from build123d import *

# Parameters (mm, degrees)
SKETCH1_W           = 8
SKETCH1_H           = 8
BOSS_EXTRUDE1_DEPTH = 8
BOSS_EXTRUDE2_DEPTH = 6
SKETCH3_OUTSIDE_W   = 19.406
SKETCH3_OUTSIDE_H   = 19.406
SKETCH3_OUTSIDE_W_2 = 10.7
SKETCH3_OUTSIDE_H_2 = 10.7
CUT_EXTRUDE2_DEPTH  = 13.354246922
CHAMFER1_SIZE       = 0.5
CHAMFER1_SIZE2      = 1.37373871
FILLET2_R           = 5
SKETCH6_W           = 8
SKETCH6_H           = 4
CUT_EXTRUDE4_DEPTH  = 12.011130732
MIRROR1_DEPTH       = 6
CUT_EXTRUDE5_DEPTH  = 10.656345064


# Read off the part's stored shape, not the designer's step: Mirror1
with BuildPart() as part:
    # Sketch1 → Boss-Extrude1 (new body)
    with BuildSketch(Plane(origin=(0, 0, 0), x_dir=(1, 0, 0), z_dir=(0, 1, 0))):
        Polygon((6.656854249, -2.757359313), (6.656854249, 2.757359313), (2.757359313, 6.656854249), (-2.757359313, 6.656854249), (-6.656854249, 2.757359313), (-6.656854249, -2.757359313), (-2.757359313, -6.656854249), (2.757359313, -6.656854249), align=None)
        Rectangle(SKETCH1_W, SKETCH1_H, mode=Mode.SUBTRACT)
    extrude(amount=BOSS_EXTRUDE1_DEPTH)

    # Sketch2 → Boss-Extrude2 (add)
    with BuildSketch(Plane.XZ):
        with BuildLine():
            Line((1, 2), (3, 4))
            Line((3, 4), (1.8, 4))
            ThreePointArc((1.8, 4), (0, 2.2), (-1.8, 4))
            Line((-1.8, 4), (-3, 4))
            Line((-3, 4), (-1, 2))
            Line((-1, 2), (-1, -4))
            Line((-1, -4), (1, -4))
            Line((1, -4), (1, 2))
        make_face()
    extrude(amount=-BOSS_EXTRUDE2_DEPTH)

    # Sketch3 outside → Cut-Extrude2 (cut, through all)
    with BuildSketch(Plane(origin=(0, 8, 0), x_dir=(1, 0, 0), z_dir=(0, 1, 0))):
        Rectangle(SKETCH3_OUTSIDE_W, SKETCH3_OUTSIDE_H)
        Rectangle(SKETCH3_OUTSIDE_W_2, SKETCH3_OUTSIDE_H_2, mode=Mode.SUBTRACT)
    extrude(amount=-CUT_EXTRUDE2_DEPTH, mode=Mode.SUBTRACT)

    # Chamfer1
    chamfer1_edges = [part.edges().sort_by_distance(p)[0] for p in [
        (-4.707106781, 0, 4.707106781),
        (-4.707106781, 0, -4.707106781),
        (4.707106781, 0, -4.707106781),
        (4.707106781, 0, 4.707106781),
        (5.35, 0, 0),
        (0, 0, -5.35),
        (-5.35, 0, 0),
        (0, 0, 5.35),
    ]]
    chamfer1_side = [part.faces().sort_by_distance(p)[0] for p in [
        (0, 0, -0.050506984),
    ]]
    chamfer(chamfer1_edges, length=CHAMFER1_SIZE, length2=CHAMFER1_SIZE2, reference=chamfer1_side[0])

    # Fillet2
    fillet2_edges = [part.edges().sort_by_distance(p)[0] for p in [
        (-1, 3, 2),
        (1, 3, 2),
    ]]
    fillet(fillet2_edges, radius=FILLET2_R)

    # Sketch6 → Cut-Extrude4 (cut, through all)
    with BuildSketch(Plane(origin=(0, 8, 0), x_dir=(1, 0, 0), z_dir=(0, 1, 0))):
        with Locations((0, 2)):
            Rectangle(SKETCH6_W, SKETCH6_H)
    extrude(amount=-CUT_EXTRUDE4_DEPTH, mode=Mode.SUBTRACT)

    # Mirror1 outline → Mirror1 (add)
    with BuildSketch(Plane(origin=(0, 0, 0), x_dir=(1, 0, 0), z_dir=(0, 1, 0))):
        with BuildLine():
            Line((-3, 4), (-2.463953695, 3.463953695))
            ThreePointArc((-2.463953695, 3.463953695), (-1.39390492, 1.874854522), (-1, 0))
            Line((-1, 0), (1, 0))
            ThreePointArc((1, 0), (1.39390492, 1.874854522), (2.463953695, 3.463953695))
            Line((2.463953695, 3.463953695), (3, 4))
            Line((3, 4), (1.8, 4))
            ThreePointArc((1.8, 4), (0, 2.2), (-1.8, 4))
            Line((-1.8, 4), (-3, 4))
        make_face()
        with BuildLine():
            Line((1, -4), (1, -2.503337045))
            ThreePointArc((1, -2.503337045), (0, -2.2), (-1, -2.503337045))
            Line((-1, -2.503337045), (-1, -4))
            Line((-1, -4), (1, -4))
        make_face()
    extrude(amount=MIRROR1_DEPTH)

    # Sketch8 → Cut-Extrude5 (cut, through all)
    with BuildSketch(Plane(origin=(0, 6, 0), x_dir=(1, 0, 0), z_dir=(0, 1, 0))):
        with BuildLine():
            Line((1.8, -4), (-1.8, -4))
            ThreePointArc((-1.8, -4), (0, -2.2), (1.8, -4))
        make_face()
    extrude(amount=-CUT_EXTRUDE5_DEPTH, mode=Mode.SUBTRACT)


solid = part.part
Geometry check sheet. Reference: the model listing, model coordinates, mm. A direction names the side the tool comes from. Give positions to 0.01 mm unless a question says otherwise; leave off trailing zeros. Write each loop counter-clockwise with the first axis right and the second up, starting at its lowest first coordinate (ties: lowest second). Pieces come first, ordered by that corner, then holes.
1) Go/stop test with a flat-tipped pin: pin 1 Ø1.5 at (x, z) = (-0.5, 3) entering from +Y. Record where the tip stops, or that it passes through.
Values follow:
pin 1: stops at y = 6
2) Cross-section at A-A (x = 0). Record the boundary of the cut face in (y, z), plus the area to 3 significant figures.
Values follow:
outline: (0, -4.85) - (1.37, -5.35) - (8, -5.35) - (8, -4) - (0, -4) - close; (0, -2.2) - (6, -2.2) - (6, 2.2) - (0, 2.2) - close; (0, 4) - (8, 4) - (8, 5.35) - (1.37, 5.35) - (0, 4.85) - close
area: 47.3 mm2
3) Set-up check for faces 1 (the face through (-4.4, 8, 0)), 2 (the face through (-1.404, 2.958, -1.9)): record each of +Z, -Z, +X, -X, +Y, -Y from which the full face is reachable in a straight line by a thin tool's end or side.
Values follow:
face 1: +Z, -Z, +X, -X, +Y
face 2: +Y, -Y
4) Thickness scan on line 1 (Z direction, x = -2, y = 7); line 2 (X direction, y = 2, z = -3.5); line 3 (X direction, y = 4.75, z = 2.75). Record the ranges inside material, lowest first.
Values follow:
line 1: z = -5.35 to -4, 4 to 5.35
line 2: x = -5.35 to -4, -2.5 to -1.73, 1.73 to 2.5, 4 to 5.35
line 3: x = -5.35 to -4, -1.87 to -1.3, 1.3 to 1.87, 4 to 5.35
5) Release check for a two-part mould opening along X. For faces 3 (the face through (-5.103, 0.696, 0.057)), 4 (the face through (4, 4, 0)), 5 (the face through (1.405, 3.042, 1.9)), 6 (the face through (0, 5, 5.35)) record: released by +X, released by -X, zero draft, split by the parting line, or undercut.
Values follow:
face 3: released by -X
face 4: undercut
face 5: undercut
face 6: zero draft
6) Cross-section at C-C (x = 3.5). Record the boundary of the cut face in (y, z).
Values follow:
outline: (0, -4.85) - (1.37, -5.35) - (8, -5.35) - (8, -4) - (0, -4) - close; (0, 4) - (8, 4) - (8, 5.35) - (1.37, 5.35) - (0, 4.85) - close
7) Cross-section at D-D (y = 6.75). Record the boundary of the cut face in (x, z).
Values follow:
outline: (-5.35, -4.06) - (-4.06, -5.35) - (4.06, -5.35) - (5.35, -4.06) - (5.35, 4.06) - (4.06, 5.35) - (-4.06, 5.35) - (-5.35, 4.06) - close; hole (-4, -4) - (4, -4) - (4, 4) - (-4, 4) - close
